Autodesk Inventor part; units mm, degrees
ref_plane "YZ Plane" through (0, 0, 0) normal (1, 0, 0) x (0, 1, 0)
ref_plane "XZ Plane" through (0, 0, 0) normal (0, 1, 0) x (-1, 0, 0)
ref_plane "XY Plane" through (0, 0, 0) normal (0, 0, 1) x (1, 0, 0)
sketch "Sketch1" plane through (0, 0, 0) normal (0, 0, 1) x (1, 0, 0)
  line L0 (0, 0) -> (3.81, 0)
  line L1 (3.81, 0) -> (3.81, -2.2225)
  line L2 (3.81, -2.2225) -> (1.905, -2.2225)
  line L3 (1.905, -2.2225) -> (1.905, -7.9375)
  line L4 (1.905, -7.9375) -> (0, -7.9375)
  line L5 (0, -7.9375) -> (0, 0)
  line L6 (0, 0) -> (0, -14.1407)
  dimension "d0" = 3.81
  dimension "d1" = 2.2225
  dimension "d2" = 1.905
  dimension "d3" = 5.715
  dimension "d4" = 90
revolve "Revolution1" add sketch "Sketch1" angle 360 about axis through (0, 0, 0) along (0, -1, 0)
chamfer "Chamfer1" distance 0.635 angle 45 1 edges at (-3.81, 0, 0)
fillet "Fillet1" radius 0.635 3 edges at (-3.175, 0, 0) (-3.81, -0.635, 0) (-3.81, -2.2225, 0)
thread "Thread1"
sketch "Sketch2" plane through (0, 0, 0) normal (0, 1, 0) x (1, 0, 0)
  line L0 (-0.752, -2.3428) -> (0.8388, -2.3428)
  line L1 (0.8388, 2.4875) -> (-0.752, 2.4875)
  line L2 (2.4007, -0.7809) -> (2.4007, 0.8966)
  line L3 (-2.3428, 0.8966) -> (-2.3428, -0.7809)
  line L4 (-2.3428, -0.7809) -> (-0.752, -0.7809)
  line L5 (0.8388, -0.7809) -> (2.4007, -0.7809)
  line L6 (2.4007, 0.8966) -> (0.8388, 0.8966)
  line L7 (-0.752, 0.8966) -> (-2.3428, 0.8966)
  line L8 (-0.752, 2.4875) -> (-0.752, 0.8966)
  line L9 (-0.752, -0.7809) -> (-0.752, -2.3428)
  line L10 (0.8388, -2.3428) -> (0.8388, -0.7809)
  line L11 (0.8388, 0.8966) -> (0.8388, 2.4875)
  point P0 (0, 0)
extrude "Extrusion1" cut sketch "Sketch2" against normal blind 1.27
properties part number "sqrew base" material "Aluminum 6061"
Work out the finished part from the listing and answer in its coordinate system (mm). A direction names the side the tool comes from. Coordinates: 2 decimals unless noted, no trailing zeros. Loops run counter-clockwise (first coordinate to the right, second up) from the corner with the lowest first, then second, coordinate; pieces in that order, holes last.
1) For faces 5 (the flat face through (0, -7.938, 0)), 6 (the flat face through (-2.343, -1, 0)), determine the directions among +Z, -Z, +X, -X, +Y, -Y from which every point of the face is accessible in a straight line to the end or side of a thin tool.
Results:
face 5: +Z, -Z, +X, -X, -Y
face 6: +Y
2) Flat-ended cylindrical pins translate along their axes: pin 1 (1 mm diameter, centred on y = -0.5, z = 2, fed in from +X); pin 2 (1 mm diameter, centred on y = -1, z = 1.5, fed in from -X); pin 3 (1 mm diameter, centred on x = 0.5, y = -0.5, fed in from -Z). Find the tip coordinate at first contact, or state that the pin passes through.
Results:
pin 1: stops at x = 3.45
pin 2: stops at x = -3.68
pin 3: stops at z = -3.81
3) Consider probe 1 along Y at (x, z) = (1.5, 0.75); probe 2 along Y at (x, z) = (1, 2.25); probe 3 along Z at (x, y) = (1.25, -5.5). Determine where each line is inside the solid, lowest interval first.
Results:
probe 1: y = -7.94 to -1.27
probe 2: y = -2.22 to 0
probe 3: z = -1.44 to 1.44
4) For a pull along X with two mould halves and no side action, classify faces 1 (the flat face through (-2, -1, -0.897)), 2 (the cylindrical face through (-0.41, -5.12, -1.86)), 3 (the flat face through (0, -2.222, -2.1)), 4 (the flat face through (2.401, -1, 0)) as +X half, -X half, draft (parallel to the pull), parting line (faces both ways), or undercut.
Results:
face 1: undercut
face 2: parting line
face 3: draft
face 4: undercut
5) Section A-A (y = -3.75) is taken. Give the vertices of the cut face in (x, z) (3 decimals).
Results:
outline: circle Ø3.81 at (0, 0)
